Model file for the job. Use its own axes, mm. Face numbers are marked on the shaded views. A direction names the side the tool comes from. Round coordinates to 2 decimals unless told otherwise and drop trailing zeros. Loops run counter-clockwise (first coordinate to the right, second up) from the corner with the lowest first, then second, coordinate; pieces in that order, holes last. Notation, with made-up numbers: (11.5, -28) -> (22.5, -28) arc R12 ccw to (22.5, -8) -> close; hole circle Ø3 at (-0.75, 84.25). An arc over 180 degrees is marked (long way). Use a Markdown table: item, result.
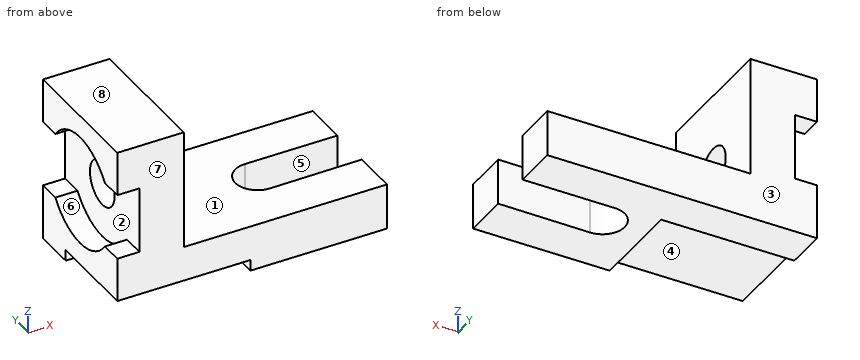
Autodesk Fusion 360 part; units mm, degrees
sketch "Sketch1" plane through (0, 0, 0) normal (0, 0, 1) x (1, 0, 0)
  line L0 (-73, -36) -> (73, -36)
  line L1 (73, -36) -> (73, 36)
  line L2 (73, 36) -> (-73, 36)
  line L3 (-73, 36) -> (-73, -36)
  line L4 (-73, -36) -> (73, 36) construction
  line L5 (73, -36) -> (-73, 36) construction
  line L6 (-73, -36) -> (-1, -36)
  line L7 (-1, -36) -> (-1, 14)
  line L8 (-1, 14) -> (-73, 14)
  line L9 (-73, 14) -> (-73, -36)
  line L10 (23.1046, -11.9995) -> (73, -11.5645)
  line L11 (23, 12) -> (73, 12)
  arc A0 (24.2094, 11.9389) -> (24.2094, -11.9389) centre (23, 0) ccw
  dimension "d1" = 146
  dimension "d2" = 72
  dimension "d3" = 72
  dimension "d4" = 50
  dimension "d5" = 24
extrude "Extrude1" add sketch "Sketch1" along normal blind 25 contours L0 L3 L6 L7 L8 L9 | L0 L1 L2 L3 L7 L8 L10 L11 A0
extrude "Extrude2" cut sketch "Sketch1" along normal blind 6 contours L0 L3 L6 L7 L8 L9
sketch "Sketch2" plane through (0, 0, 25) normal (0, 0, 1) x (-1, 0, 0)
  arc A0 (-23, -12) -> (-23.1046, 11.9995) centre (-23, 0) ccw
  line L0 (-23, -12) -> (-73, -12)
  line L1 (-73, -12) -> (-73, -36)
  line L2 (-73, -36) -> (73, -36)
  line L3 (73, -36) -> (73, 36)
  line L4 (73, 36) -> (-73, 36)
  line L5 (-73, 36) -> (-73, 11.5645)
  line L6 (-73, 11.5645) -> (-23.1046, 11.9995)
  line L7 (73, 36) -> (37, 36)
  line L8 (37, 36) -> (37, -36)
  line L9 (37, -36) -> (73, -36)
  line L10 (73, -36) -> (73, 36)
  dimension "d11" = 36
extrude "Extrude3" add sketch "Sketch2" along normal blind 65 contours L2 L3 L4 L7 L8 L9 L10
sketch "Sketch3" plane through (-73, 0, 0) normal (-1, 0, 0) x (0, -1, 0)
  line L0 (-14, 0) -> (-14, 6)
  line L1 (-14, 6) -> (36, 6)
  line L2 (36, 6) -> (36, 90)
  line L3 (36, 90) -> (-36, 90)
  line L4 (-36, 90) -> (-36, 0)
  line L5 (-36, 0) -> (-14, 0)
  circle A0 centre (0, 48) radius 12
  circle A1 centre (0, 48) radius 30
  line L6 (-36, 90) -> (36, 90)
  line L7 (36, 90) -> (36, 66)
  line L8 (36, 66) -> (-36, 66)
  line L9 (-36, 66) -> (-36, 90)
  line L10 (36, 6) -> (-36, 6)
  line L11 (-36, 6) -> (-36, 30)
  line L12 (-36, 30) -> (36, 30)
  line L13 (36, 30) -> (36, 6)
  dimension "d14" = 24
  dimension "d15" = 60
  dimension "d16" = 48
  dimension "d17" = 24
  dimension "d18" = 24
extrude "Extrude4" cut sketch "Sketch3" against normal through all contours A0
extrude "Extrude5" cut sketch "Sketch3" against normal blind 12 contours L2 A1 L8 L12 | L4 A1 L8 L12 | A1 L8 L12 | A1 L12 | A1 L8
Q1. Band-saw the part on A-A, the plane y = 0. Give the cut face in (x, z), plus the area to 3 significant figures.
Results list:
| item | result |
|---|---|
| outline | (-73, 6) -> (-1, 6) -> (-1, 0) -> (11, 0) -> (11, 25) -> (-37, 25) -> (-37, 36) -> (-61, 36) -> (-61, 18) -> (-73, 18) -> close; (-73, 78) -> (-61, 78) -> (-61, 60) -> (-37, 60) -> (-37, 90) -> (-73, 90) -> close |
| area | 2,710 mm² |
Q2. Pull direction Y, two halves, no side cores. Call the marked faces 5, 6, 7 and 8: released by +Y, released by -Y, zero draft, split by the parting line, or undercut.
Results list:
| item | result |
|---|---|
| face 5 | undercut |
| face 6 | undercut |
| face 7 | released by -Y |
| face 8 | zero draft |
Q3. Band-saw the part on C-C, the plane y = -26.5. Give the cut face in (x, z), plus the area to 3 significant figures.
Results list:
| item | result |
|---|---|
| outline | (-73, 6) -> (-1, 6) -> (-1, 0) -> (73, 0) -> (73, 25) -> (-37, 25) -> (-37, 90) -> (-73, 90) -> (-73, 66) -> (-61, 66) -> (-61, 30) -> (-73, 30) -> close |
| area | 5,130 mm² |
Q4. Flat gauge pins, fed straight in: pin 1 (3 mm diameter, centred on y = 8.5, z = 62.5, fed in from -X); pin 2 (14.5 mm diameter, centred on y = 0, z = 48, fed in from +X); pin 3 (6 mm diameter, centred on x = 55.5, y = -24, fed in from +Z); pin 4 (1 mm diameter, centred on y = 5, z = 13.5, fed in from +X). Where does each tip first touch, or does it go through?
Results list:
| item | result |
|---|---|
| pin 1 | stops at x = -61 |
| pin 2 | passes through |
| pin 3 | stops at z = 25 |
| pin 4 | stops at x = 12.33 |
Q5. Band-saw the part on D-D, the plane x = -9. Give the cut face in (y, z).
Results list:
| item | result |
|---|---|
| outline | (-36, 6) -> (14, 6) -> (14, 0) -> (36, 0) -> (36, 25) -> (-36, 25) -> close |
Q6. Band-saw the part on B-B, the plane z = 48. Give the cut face in (x, y).
Results list:
| item | result |
|---|---|
| outline | (-61, -36) -> (-37, -36) -> (-37, -12) -> (-61, -12) -> close; (-61, 12) -> (-37, 12) -> (-37, 36) -> (-61, 36) -> close |
Q7. Drill centre lines: L1, parallel to Z at x = -49, y = 0; L2, parallel to X at y = -24.5, z = 56; L3, parallel to X at y = 20, z = 73.5. Where is each one in solid material? Low to high. Write a range as from..to.
Results list:
| item | result |
|---|---|
| L1 | z = 6..36, 60..90 |
| L2 | x = -61..-37 |
| L3 | x = -73..-37 |
Q8. Tool access for the marked faces 1, 2, 3 and 4: list every direction of +Z, -Z, +X, -X, +Y, -Y with a clear straight run to the whole face (end or side of a thin tool).
Results list:
| item | result |
|---|---|
| face 1 | +Z, +X, +Y, -Y |
| face 2 | -X |
| face 3 | +Z, -Z, +X, -X, +Y |
| face 4 | -Z, -X, -Y |
